```python
from build123d import *

# Parameters (mm, degrees)
SKETCH1_R                    = 50
BOSS_EXTRUDE1_DEPTH          = 5
F_10_2_10_2_DIAMETER_HOLE1_D = 10.2
M3_CLEARANCE_HOLE1_D         = 3.4
SKETCH9_R                    = 7.5
CUT_EXTRUDE1_DEPTH           = 10
SKETCH10_R                   = 1.5
CUT_EXTRUDE2_DEPTH           = 10
SKETCH11_R                   = 4
CUT_EXTRUDE3_DEPTH           = 10


with BuildPart() as part:
    # Sketch1 → Boss-Extrude1 (new body)
    with BuildSketch(Plane.XY):
        Circle(SKETCH1_R)
    extrude(amount=BOSS_EXTRUDE1_DEPTH)

    # Ø10.2 (10.2) Diameter Hole1 (through all)
    with Locations(Plane(origin=(0, 0, 0), x_dir=(-1, 0, 0), z_dir=(0, 0, -1))):
        with Locations((37, 0), (-37, 0), (0, -40)):
            Hole(F_10_2_10_2_DIAMETER_HOLE1_D / 2)

    # M3 Clearance Hole1 (through all)
    with Locations(Plane.XY.offset(5)):
        with Locations((46, 0), (28, 0), (9, -40), (-9, -40), (-46, 0), (-28, 0)):
            Hole(M3_CLEARANCE_HOLE1_D / 2)

    # Sketch9 → Cut-Extrude1 (cut)
    with BuildSketch(Plane.XY.offset(5)):
        with Locations((0, 26)):
            Circle(SKETCH9_R)
    extrude(amount=-CUT_EXTRUDE1_DEPTH, mode=Mode.SUBTRACT)

    # Sketch10 → Cut-Extrude2 (cut)
    with BuildSketch(Plane.XY.offset(5)):
        with Locations((10, -9)):
            Circle(SKETCH10_R)
        with Locations((-10, -9)):
            Circle(SKETCH10_R)
        with BuildLine():
            Line((-19, -13), (19, -13))
            ThreePointArc((19, -13), (20.414213562, -13.585786438), (21, -15))
            Line((21, -15), (21, -23))
            ThreePointArc((21, -23), (20.414213562, -24.414213562), (19, -25))
            Line((19, -25), (-19, -25))
            ThreePointArc((-19, -25), (-20.414213562, -24.414213562), (-21, -23))
            Line((-21, -23), (-21, -15))
            ThreePointArc((-21, -15), (-20.414213562, -13.585786438), (-19, -13))
        make_face()
    extrude(amount=-CUT_EXTRUDE2_DEPTH, mode=Mode.SUBTRACT)

    # Sketch11 → Cut-Extrude3 (cut)
    with BuildSketch(Plane.XY.offset(5)):
        with Locations((-39.87754263, -18.595203517)):
            Circle(SKETCH11_R)
        with Locations((39.87754263, -18.595203517)):
            Circle(SKETCH11_R)
    extrude(amount=-CUT_EXTRUDE3_DEPTH, mode=Mode.SUBTRACT)


solid = part.part
```
Design review of the part built by this model. Coordinates are the model's own, in mm. Coordinates: 2 decimals unless noted, no trailing zeros. Loops run counter-clockwise (first coordinate to the right, second up) from the corner with the lowest first, then second, coordinate; pieces in that order, holes last.
Q1. For pin 1 (9 mm diameter, centred on x = -39.88, y = -18.6, fed in from +Z); pin 2 (1.5 mm diameter, centred on y = 2, z = 3, fed in from -X); pin 3 (1.5 mm diameter, centred on y = -6.5, z = 3.5, fed in from +X); pin 4 (3 mm diameter, centred on x = 13.5, z = 4, fed in from -Y), all flat-tipped, find the tip position at first contact; note any pin that passes through.
Reported:
pin 1: stops at z = 5
pin 2: stops at x = -49.98
pin 3: stops at x = 49.67
pin 4: stops at y = -48.54
Q2. To check wall thickness, follow line 1 (X direction, y = -10, z = 1.35); line 2 (X direction, y = -39, z = 0.55); line 3 (X direction, y = -17, z = 3.5). State the ranges of each line that lie inside material, in increasing order.
Reported:
line 1: x = -48.99 to -11.12, -8.88 to 8.88, 11.12 to 48.99
line 2: x = -31.29 to -10.37, -7.63 to -5, 5 to 7.63, 10.37 to 31.29
line 3: x = -47.02 to -43.55, -36.21 to -21, 21 to 36.21, 43.55 to 47.02
Q3. The part is to be moulded in two halves that separate along X. For faces 1 (the face through (-1, 1, 0)), 2 (the face through (47.69, 15.02, 2.46)), 3 (the face through (-11.2, -9.9, 2.5)), say which applies: +X half, -X half, draft (parallel to the pull), parting line (faces both ways), or undercut.
Reported:
face 1: draft
face 2: parting line
face 3: undercut
Q4. We need section B-B on y = -9. State the section outline as (x, z) points, and give its area (3 significant figures).
Reported:
outline: (-49.18, 0) - (-11.5, 0) - (-11.5, 5) - (-49.18, 5) - close; (-8.5, 0) - (8.5, 0) - (8.5, 5) - (-8.5, 5) - close; (11.5, 0) - (49.18, 0) - (49.18, 5) - (11.5, 5) - close
area: 462 mm2
Q5. We need section D-D on x = -28. State the section outline as (y, z) points.
Reported:
outline: (-41.42, 0) - (-1.7, 0) - (-1.7, 5) - (-41.42, 5) - close; (1.7, 0) - (41.42, 0) - (41.42, 5) - (1.7, 5) - close
Q6. We need section C-C on z = 4. State how many separate pieces and enclosed holes the cut face has, and give its area (3 significant figures).
Reported:
separate pieces: 1
enclosed holes: 15
area: 6,760 mm2
Q7. We need section A-A on x = 39. State the section outline as (y, z) points, and give its area (3 significant figures).
Reported:
outline: (-31.29, 0) - (-22.5, 0) - (-22.5, 5) - (-31.29, 5) - close; (-14.69, 0) - (-4.69, 0) - (-4.69, 5) - (-14.69, 5) - close; (4.69, 0) - (31.29, 0) - (31.29, 5) - (4.69, 5) - close
area: 227 mm2
